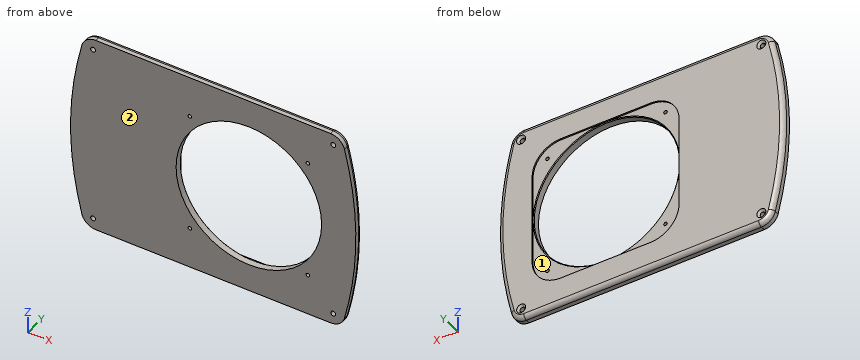
from build123d import *

# Parameters (mm, degrees)
BOSS_EXTRUDE1_DEPTH                             = 6
FILLET1_R                                       = 10
FILLET2_R                                       = 3
CUT_EXTRUDE1_REACH                              = 124.213
SKETCH2_R                                       = 51
M3X0_5_TAPPED_HOLE1_D                           = 2.5
CSK_FOR_M3_FLAT_HEAD_MACHINE_SCREW6_D           = 3.4
CSK_FOR_M3_FLAT_HEAD_MACHINE_SCREW6_CSINK_D     = 6.3
CSK_FOR_M3_FLAT_HEAD_MACHINE_SCREW6_CSINK_ANGLE = 90
SKETCH2_7_W                                     = 103
SKETCH2_7_H                                     = 103
CUT_EXTRUDE3_DEPTH                              = 1
FILLET4_R                                       = 20
CHAMFER1_SIZE                                   = 0.5


with BuildPart() as part:
    # Sketch1 → Boss-Extrude1 (new body)
    with BuildSketch(Plane(origin=(0, 0, 0), x_dir=(1, 0, 0), z_dir=(0, 1, 0))):
        with BuildLine():
            Line((-90, 70), (90, 70))
            add(Edge.make_bspline(
                [(90, 70), (110, 0), (90, -70)],
                knots=[0, 0, 0, 1, 1, 1], degree=2))
            Line((90, -70), (-90, -70))
            add(Edge.make_bspline(
                [(-90, 70), (-110, 0), (-90, -70)],
                knots=[0, 0, 0, 1, 1, 1], degree=2))
        make_face()
    extrude(amount=BOSS_EXTRUDE1_DEPTH)

    # Fillet1
    fillet1_edges = [part.edges().sort_by_distance(p)[0] for p in [
        (-90, 3, -70),
        (90, 3, -70),
        (90, 3, 70),
        (-90, 3, 70),
    ]]
    fillet(fillet1_edges, radius=FILLET1_R)

    # Fillet2
    fillet2_edges = [part.edges().sort_by_distance(p)[0] for p in [
        (-100, 6, -3e-09),
        (0, 6, -70),
        (100, 6, -3e-09),
        (0, 6, 70),
        (-88.48120263, 6, 67.896446056),
        (88.48120263, 6, 67.896446056),
        (88.48120263, 6, -67.896446056),
        (-88.48120263, 6, -67.896446056),
    ]]
    fillet(fillet2_edges, radius=FILLET2_R)

    # Sketch2 → Cut-Extrude1 (cut, up to next)
    with BuildSketch(Plane(origin=(0, 6, 0), x_dir=(1, 0, 0), z_dir=(0, 1, 0)), mode=Mode.PRIVATE) as cut_extrude1_sk1:
        with Locations(Location((25, 0, 0), (0, 0, 270))):
            Circle(SKETCH2_R)
    cut_extrude1_tool1 = extrude(cut_extrude1_sk1.sketch, amount=-CUT_EXTRUDE1_REACH, mode=Mode.PRIVATE) & part.part
    add(cut_extrude1_tool1.solids().sort_by_distance((25, 6, 0))[0], mode=Mode.SUBTRACT)

    # M3x0.5 Tapped Hole1 (through all)
    with Locations(Plane(origin=(0, 6, 0), x_dir=(1, 0, 0), z_dir=(0, 1, 0))):
        with Locations((66.365746699, 41.365746699), (66.365746699, -41.365746699), (-16.365746699, -41.365746699), (-16.365746699, 41.365746699)):
            Hole(M3X0_5_TAPPED_HOLE1_D / 2)

    # CSK for M3 Flat Head Machine Screw6 (through all)
    with Locations(Plane(origin=(0, 6, 0), x_dir=(1, 0, 0), z_dir=(0, 1, 0))):
        with Locations((-84.186251123, 62.368933817), (84.186251123, 62.368933817), (84.186251123, -62.368933817), (-84.186251123, -62.368933817)):
            CounterSinkHole(CSK_FOR_M3_FLAT_HEAD_MACHINE_SCREW6_D / 2, CSK_FOR_M3_FLAT_HEAD_MACHINE_SCREW6_CSINK_D / 2, counter_sink_angle=CSK_FOR_M3_FLAT_HEAD_MACHINE_SCREW6_CSINK_ANGLE)

    # Sketch2<7> → Cut-Extrude3 (cut)
    with BuildSketch(Plane(origin=(0, 6, 0), x_dir=(1, 0, 0), z_dir=(0, 1, 0))):
        with Locations((25, 0)):
            Rectangle(SKETCH2_7_W, SKETCH2_7_H)
    extrude(amount=-CUT_EXTRUDE3_DEPTH, mode=Mode.SUBTRACT)

    # Fillet4
    fillet4_edges = [part.edges().sort_by_distance(p)[0] for p in [
        (76.5, 5.5, 51.5),
        (-26.5, 5.5, 51.5),
        (-26.5, 5.5, -51.5),
        (76.5, 5.5, -51.5),
    ]]
    fillet(fillet4_edges, radius=FILLET4_R)

    # Chamfer1
    chamfer1_edges = [part.edges().sort_by_distance(p)[0] for p in [
        (25, 5, -51),
    ]]
    chamfer(chamfer1_edges, length=CHAMFER1_SIZE - 0.0001)  # a hair under: the kernel refuses the full size


solid = part.part
CAD build for the part. Positions are in the model's coordinates, mm. Face numbers are marked on the shaded views. Coordinates: 2 decimals unless noted, no trailing zeros. Return JSON: item names as keys, results as strings.
Item 1: Probe line 1 (X direction, y = 2.35, z = 0); line 2 (Z direction, x = -84, y = 3.25); line 3 (X direction, y = 1.75, z = -30.5). List the from-to ranges inside material, lowest first. Write a range as from..to.
Findings below:
{"line 1": "x = -100..-26, 76..100", "line 2": "z = -69.85..-64.06, -60.68..60.68, 64.06..69.85", "line 3": "x = -98.1..-15.87, 65.87..98.1"}
Item 2: Two-plate mould, pull along Z, no slides. Class the marked faces 1 and 2: +Z half, -Z half, draft (parallel to the pull), parting line (faces both ways), or undercut.
Findings below:
{"face 1": "undercut", "face 2": "draft"}
Item 3: Drop flat-ended pins along their axis: pin 1 Ø5.5 at (x, z) = (-84.19, 62.37) entering from +Y; pin 2 Ø1.5 at (x, z) = (66.37, 41.37) entering from +Y; pin 3 Ø3 at (x, z) = (66.37, -41.37) entering from +Y; pin 4 Ø2 at (y, z) = (2.5, 9.5) entering from +X. Give the stop position or say it passes through.
Findings below:
{"pin 1": "stops at y = 5.6", "pin 2": "passes through", "pin 3": "stops at y = 5", "pin 4": "stops at x = 99.85"}
